Could you check a few things on this model? Use its own coordinates, in mm. Coordinates: 2 decimals unless noted, no trailing zeros. Loops run counter-clockwise (first coordinate to the right, second up) from the corner with the lowest first, then second, coordinate; pieces in that order, holes last. Notation, with made-up numbers: (31.25, 86.25) -> (51.25, 86.25) arc R21 cw to (51.25, 122.25) -> close; hole circle Ø10 at (-24.75, 72). An arc over 180 degrees is marked (long way). One line per question, with ' | ' between items.
```python
from build123d import *

# Parameters (mm, degrees)
F1_DEPTH = 3.175
F3_DEPTH = 3.175


with BuildPart() as f1:
    # F0 (on Top) → F1 (new body)
    with BuildSketch(Plane.XY):
        with BuildLine():
            Line((168.37406, 139.7), (-307.8226, 139.7))
            ThreePointArc((-307.8226, 139.7), (-314.557792, 136.910192), (-317.3476, 130.175))
            Line((-317.3476, 130.175), (-317.3476, -3.175))
            ThreePointArc((-317.3476, -3.175), (-314.557792, -9.910192), (-307.8226, -12.7))
            Line((-307.8226, -12.7), (168.37406, -12.7))
            ThreePointArc((168.37406, -12.7), (175.109252, -9.910192), (177.89906, -3.175))
            Line((177.89906, -3.175), (177.89906, 130.175))
            ThreePointArc((177.89906, 130.175), (175.109252, 136.910192), (168.37406, 139.7))
        make_face()
        with BuildLine():
            ThreePointArc((0, 9.525), (-2.789808, 2.789808), (-9.525, 0))
            Line((-9.525, 0), (-117.475, 0))
            ThreePointArc((-117.475, 0), (-124.210192, 2.789808), (-127, 9.525))
            Line((-127, 9.525), (-127, 117.475))
            ThreePointArc((-127, 117.475), (-124.210192, 124.210192), (-117.475, 127))
            Line((-117.475, 127), (-9.525, 127))
            ThreePointArc((-9.525, 127), (-2.789808, 124.210192), (0, 117.475))
            Line((0, 117.475), (0, 9.525))
        make_face(mode=Mode.SUBTRACT)
    extrude(amount=F1_DEPTH)

    # F2 (on face) → F3 (join)
    with BuildSketch(Plane.XY.offset(3.175)):
        with BuildLine():
            Line((171.54906, 152.4), (-120.65, 152.4))
            ThreePointArc((-120.65, 152.4), (-125.140128, 150.540128), (-127, 146.05))
            Line((-127, 146.05), (-127, 127))
            Line((-127, 127), (-9.525, 127))
            ThreePointArc((-9.525, 127), (-2.789808, 124.210192), (0, 117.475))
            Line((0, 117.475), (0, 9.525))
            ThreePointArc((0, 9.525), (-2.789808, 2.789808), (-9.525, 0))
            Line((-9.525, 0), (-127, 0))
            Line((-127, 0), (-127, -19.05))
            ThreePointArc((-127, -19.05), (-125.140128, -23.540128), (-120.65, -25.4))
            Line((-120.65, -25.4), (171.54906, -25.4))
            ThreePointArc((171.54906, -25.4), (176.039188, -23.540128), (177.89906, -19.05))
            Line((177.89906, -19.05), (177.89906, 146.05))
            ThreePointArc((177.89906, 146.05), (176.039188, 150.540128), (171.54906, 152.4))
        make_face()
    extrude(amount=F3_DEPTH)


solid = f1.part
```
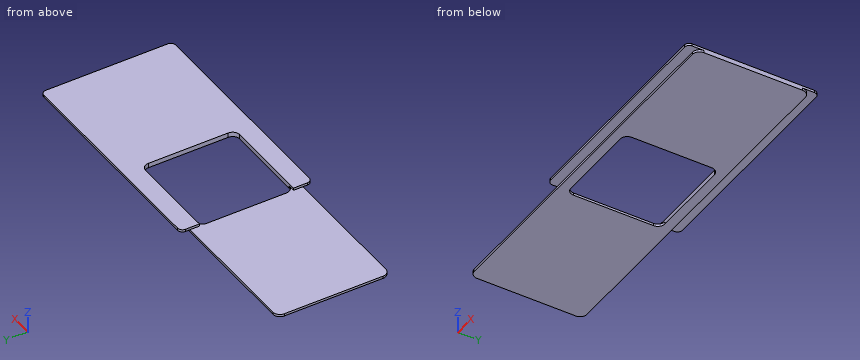
Q1. Imagine slicing it at D-D on x = 137. Write out the boundary of the cut face in (y, z) (3 decimals).
Values follow:
outline: (-25.4, 3.175) -> (-12.7, 3.175) -> (-12.7, 0) -> (139.7, 0) -> (139.7, 3.175) -> (152.4, 3.175) -> (152.4, 6.35) -> (-25.4, 6.35) -> close
Q2. Please list where these lines run through material, in increasing order: L1, parallel to X at y = 98.5, z = 1; L2, parallel to Y at x = -105, z = 3.5; L3, parallel to X at y = 66, z = 5.25. Write a range as [from, to].
Values follow:
L1: x = [-317.35, -127], [0, 177.9] | L2: y = [-25.4, 0], [127, 152.4] | L3: x = [0, 177.9]
Q3. For pin 1 (6 mm diameter, centred on x = 22, y = 49.5, fed in from -Z); pin 2 (1 mm diameter, centred on y = 137.5, z = 5.5, fed in from -X); pin 3 (3 mm diameter, centred on x = -197.5, z = 4, fed in from +Y); pin 4 (1.6 mm diameter, centred on x = -105, z = 1, fed in from -Y), each with a flat end and sliding along its axis, tell me the tip position at first contact or that it passes through.
Values follow:
pin 1: stops at z = 0 | pin 2: stops at x = -127 | pin 3: stops at y = 139.7 | pin 4: stops at y = -12.7
Q4. Imagine slicing it at B-B on y = 83. Write out the boundary of the cut face in (x, z) (3 decimals), plus the area to 3 significant figures.
Values follow:
outline: (-317.348, 0) -> (-127, 0) -> (-127, 3.175) -> (-317.348, 3.175) -> close; (0, 0) -> (177.899, 0) -> (177.899, 6.35) -> (0, 6.35) -> close | area: 1,730 mm2
Q5. Imagine slicing it at C-C on z = 1. Write out the boundary of the cut face in (x, y) (3 decimals), plus the area to 3 significant figures.
Values follow:
outline: (-317.348, -3.175) arc R9.525 ccw to (-307.823, -12.7) -> (168.374, -12.7) arc R9.525 ccw to (177.899, -3.175) -> (177.899, 130.175) arc R9.525 ccw to (168.374, 139.7) -> (-307.823, 139.7) arc R9.525 ccw to (-317.348, 130.175) -> close; hole (-127, 9.525) arc R9.525 ccw to (-117.475, 0) -> (-9.525, 0) arc R9.525 ccw to (0, 9.525) -> (0, 117.475) arc R9.525 ccw to (-9.525, 127) -> (-117.475, 127) arc R9.525 ccw to (-127, 117.475) -> close | area: 59,300 mm2
Q6. Imagine slicing it at A-A on x = -30.5. Write out the boundary of the cut face in (y, z) (3 decimals), plus the area to 3 significant figures.
Values follow:
outline: (-25.4, 3.175) -> (-12.7, 3.175) -> (-12.7, 0) -> (0, 0) -> (0, 6.35) -> (-25.4, 6.35) -> close; (127, 0) -> (139.7, 0) -> (139.7, 3.175) -> (152.4, 3.175) -> (152.4, 6.35) -> (127, 6.35) -> close | area: 242 mm2
